```python
from build123d import *

# Parameters (mm, degrees)
SKETCH_1_W          = 40
SKETCH_1_H          = 20
SKETCH_1_W_2        = 36
SKETCH_1_H_2        = 16
EXTRUDE_1_DEPTH     = 190
SKETCH_3_R          = 2.15
SKETCH_3_R_2        = 7.5
CUT_EXTRUDE_2_DEPTH = 21
SKETCH_4_W          = 20
SKETCH_4_H          = 20
CUT_EXTRUDE_3_DEPTH = 41
SKETCH_5_R          = 2.5
CUT_EXTRUDE_4_DEPTH = 21
SKETCH_6_R          = 2.5
CUT_EXTRUDE_5_DEPTH = 21
SKETCH_7_R          = 2.65
CUT_EXTRUDE_6_DEPTH = 21
SKETCH_8_R          = 1.7
CUT_EXTRUDE_7_DEPTH = 41
SKETCH_9_R          = 2.1
SKETCH_9_R_2        = 2.15
CUT_EXTRUDE_8_DEPTH = 41


with BuildPart() as part:
    # 草图1 → 拉伸-薄壁1 (new body)
    with BuildSketch(Plane.XY):
        Rectangle(SKETCH_1_W, SKETCH_1_H)
        Rectangle(SKETCH_1_W_2, SKETCH_1_H_2, mode=Mode.SUBTRACT)
    extrude(amount=EXTRUDE_1_DEPTH)

    # 草图3 → 切除-拉伸2 (cut, through all)
    with BuildSketch(Plane(origin=(0, 10, 0), x_dir=(1, 0, 0), z_dir=(0, 1, 0))):
        with Locations((-12.5, -184.5)):
            Circle(SKETCH_3_R)
        with Locations((-12.5, -159.5)):
            Circle(SKETCH_3_R)
        with Locations((12.5, -159.5)):
            Circle(SKETCH_3_R)
        with Locations((12.5, -184.5)):
            Circle(SKETCH_3_R)
        with Locations((0, -172)):
            Circle(SKETCH_3_R_2)
    extrude(amount=-CUT_EXTRUDE_2_DEPTH, mode=Mode.SUBTRACT)

    # 草图4 → 切除-拉伸3 (cut, through all)
    with BuildSketch(Plane(origin=(20, 0, 0), x_dir=(0, 0, -1), z_dir=(1, 0, 0))):
        with Locations((-10, 0)):
            Rectangle(SKETCH_4_W, SKETCH_4_H)
    extrude(amount=-CUT_EXTRUDE_3_DEPTH, mode=Mode.SUBTRACT)

    # 草图5 → 切除-拉伸4 (cut, through all)
    with BuildSketch(Plane(origin=(0, 10, 0), x_dir=(1, 0, 0), z_dir=(0, 1, 0))):
        with Locations((0, -145)):
            Circle(SKETCH_5_R)
        with Locations((0, -85)):
            Circle(SKETCH_5_R)
        with Locations((0, -72.5)):
            Circle(SKETCH_5_R)
    extrude(amount=-CUT_EXTRUDE_4_DEPTH, mode=Mode.SUBTRACT)

    # 草图6 → 切除-拉伸5 (cut, through all)
    with BuildSketch(Plane(origin=(0, 10, 0), x_dir=(1, 0, 0), z_dir=(0, 1, 0))):
        with Locations((-14.5, -133.038475773)):
            Circle(SKETCH_6_R)
        with Locations((14.5, -133.038475773)):
            Circle(SKETCH_6_R)
        with Locations((14.5, -28.038475773)):
            Circle(SKETCH_6_R)
        with Locations((-14.5, -28.038475773)):
            Circle(SKETCH_6_R)
    extrude(amount=-CUT_EXTRUDE_5_DEPTH, mode=Mode.SUBTRACT)

    # 草图7 → 切除-拉伸6 (cut, through all)
    with BuildSketch(Plane.XZ.offset(10)):
        with Locations((-10, 45)):
            Circle(SKETCH_7_R)
        with Locations((10, 45)):
            Circle(SKETCH_7_R)
    extrude(amount=-CUT_EXTRUDE_6_DEPTH, mode=Mode.SUBTRACT)

    # 草图8 → 切除-拉伸7 (cut, through all)
    with BuildSketch(Plane(origin=(20, 0, 0), x_dir=(0, 0, -1), z_dir=(1, 0, 0))):
        with Locations((-28, 5)):
            Circle(SKETCH_8_R)
        with Locations((-28, -5)):
            Circle(SKETCH_8_R)
    extrude(amount=-CUT_EXTRUDE_7_DEPTH, mode=Mode.SUBTRACT)

    # 草图9 → 切除-拉伸8 (cut, through all)
    with BuildSketch(Plane.ZY.offset(20)):
        with Locations((63, -5)):
            Circle(SKETCH_9_R)
        with Locations((63, 5)):
            Circle(SKETCH_9_R)
        with Locations((98, 0)):
            Circle(SKETCH_9_R_2)
        with Locations((118, 0)):
            Circle(SKETCH_9_R_2)
        with Locations((138, 0)):
            Circle(SKETCH_9_R_2)
    extrude(amount=-CUT_EXTRUDE_8_DEPTH, mode=Mode.SUBTRACT)


solid = part.part
```
Check sheet for the modelled part. Datum: model origin and axes. Units: mm. A direction names the side the tool comes from. Coordinates: 2 decimals unless noted, no trailing zeros. Loops run counter-clockwise (first coordinate to the right, second up) from the corner with the lowest first, then second, coordinate; pieces in that order, holes last.
1) Sectioned sample at B-B (y = 5). Record the boundary of the cut face in (x, z), and give its area (3 significant figures).
2) Sectioned sample at C-C (z = 98). Record the boundary of the cut face in (x, y).
3) Access from +Z, -Z, +X, -X, +Y, -Y to the whole of each face (thin tool, end or side, straight path). Record for faces 5 (the face through (18.99, 0.09, 95.85)), 6 (the face through (-18, 0, 104)).
4) Gauge pin test, flat end, axial feed: pin 1 (2 mm diameter, centred on y = 5, z = 28, fed in from -X) (3 decimals). Record the tip position at first contact, or that the pin passes through.
5) Sectioned sample at A-A (z = 159.5). Record the boundary of the cut face in (x, y), and give its area (3 significant figures).
6) Release check for a two-part mould opening along Y. For faces 1 (the face through (-13.35, 9.01, 135.26)), 2 (the face through (-19.014, 5.631, 65.003)), 3 (the face through (0, 8, 104)), 4 (the face through (0, 10, 104)) record: released by +Y, released by -Y, zero draft, split by the parting line, or undercut.
7) Sectioned sample at D-D (x = -5.5). Record the boundary of the cut face in (y, z).
8) Material ranges on probe 1 along X at (y, z) = (-2, 91.5); probe 2 along Y at (x, z) = (-5, 140); probe 3 along Y at (x, z) = (-19, 98), recorded low to high.
Check sheet entries:
1. outline: (-20, 20) - (-18, 20) - (-18, 26.3) - (-20, 26.3) - close; (-20, 29.7) - (-18, 29.7) - (-18, 60.9) - (-20, 60.9) - close; (-20, 65.1) - (-18, 65.1) - (-18, 190) - (-20, 190) - close; (18, 20) - (20, 20) - (20, 26.3) - (18, 26.3) - close; (18, 29.7) - (20, 29.7) - (20, 60.9) - (18, 60.9) - close; (18, 65.1) - (20, 65.1) - (20, 190) - (18, 190) - close
1. area: 650 mm2
2. outline: (-20, -10) - (20, -10) - (20, -2.15) - (18, -2.15) - (18, -8) - (-18, -8) - (-18, -2.15) - (-20, -2.15) - close; (-20, 2.15) - (-18, 2.15) - (-18, 8) - (18, 8) - (18, 2.15) - (20, 2.15) - (20, 10) - (-20, 10) - close
3. face 5: +X, -X
3. face 6: +Z, -Z
4. pin 1: passes through
5. outline: (-20, -10) - (-14.65, -10) - (-14.65, -8) - (-18, -8) - (-18, 8) - (-14.65, 8) - (-14.65, 10) - (-20, 10) - close; (-10.35, -10) - (10.35, -10) - (10.35, -8) - (-10.35, -8) - close; (-10.35, 8) - (10.35, 8) - (10.35, 10) - (-10.35, 10) - close; (14.65, -10) - (20, -10) - (20, 10) - (14.65, 10) - (14.65, 8) - (18, 8) - (18, -8) - (14.65, -8) - close
5. area: 190 mm2
6. face 1: zero draft
6. face 2: undercut
6. face 3: undercut
6. face 4: released by +Y
7. outline: (-10, 20) - (-8, 20) - (-8, 166.9) - (-10, 166.9) - close; (-10, 177.1) - (-8, 177.1) - (-8, 190) - (-10, 190) - close; (8, 20) - (10, 20) - (10, 166.9) - (8, 166.9) - close; (8, 177.1) - (10, 177.1) - (10, 190) - (8, 190) - close
8. probe 1: x = -20 to -18, 18 to 20
8. probe 2: y = -10 to -8, 8 to 10
8. probe 3: y = -10 to -2.15, 2.15 to 10
